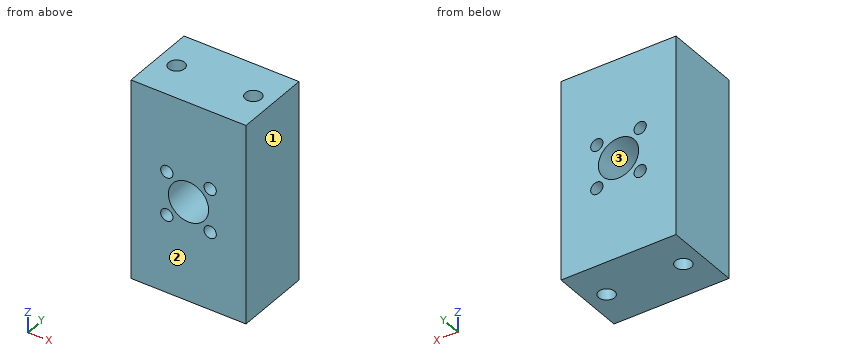
```python
from build123d import *

# Parameters (mm, degrees)
SKETCH_1_W          = 30
SKETCH_1_H          = 20
SKETCH_1_R          = 2.1
EXTRUDE_1_DEPTH     = 52
SKETCH_2_R          = 5.25
SKETCH_2_R_2        = 1.6
CUT_EXTRUDE_1_DEPTH = 64.277168078


with BuildPart() as part:
    # 草图1 → 凸台-拉伸1 (new body)
    with BuildSketch(Plane.XY):
        with Locations((15, 10)):
            Rectangle(SKETCH_1_W, SKETCH_1_H)
        with Locations(Location((5, 10, 0), (0, 0, 180))):
            Circle(SKETCH_1_R, mode=Mode.SUBTRACT)
        with Locations(Location((25, 10, 0), (0, 0, 180))):
            Circle(SKETCH_1_R, mode=Mode.SUBTRACT)
    extrude(amount=EXTRUDE_1_DEPTH)

    # 草图2 → 切除-拉伸1 (cut, through all)
    with BuildSketch(Plane(origin=(0, 20, 0), x_dir=(1, 0, 0), z_dir=(0, 1, 0))):
        with Locations(Location((15, -26, 0), (0, 0, 270))):
            Circle(SKETCH_2_R)
        with Locations(Location((9.343145751, -31.656854249, 0), (0, 0, 270))):
            Circle(SKETCH_2_R_2)
        with Locations(Location((9.343145751, -20.343145751, 0), (0, 0, 270))):
            Circle(SKETCH_2_R_2)
        with Locations(Location((20.656854249, -20.343145751, 0), (0, 0, 270))):
            Circle(SKETCH_2_R_2)
        with Locations(Location((20.656854249, -31.656854249, 0), (0, 0, 270))):
            Circle(SKETCH_2_R_2)
    extrude(amount=-CUT_EXTRUDE_1_DEPTH, mode=Mode.SUBTRACT)


solid = part.part
```
Input: part model. Units: mm. Frame: model coordinates. Face numbers are marked on the shaded views. Round coordinates to 2 decimals unless told otherwise and drop trailing zeros. Loops run counter-clockwise (first coordinate to the right, second up) from the corner with the lowest first, then second, coordinate; pieces in that order, holes last. Notation, with made-up numbers: (23, 2) -> (44, 2) arc R21 ccw to (44, 20) -> close; hole circle Ø11 at (-4, 6.5). An arc over 180 degrees is marked (long way). Use one line per item in the form item = value. Start each with the question number.
Item 1: Material intervals for L1, parallel to X at y = 10, z = 14; L2, parallel to X at y = 18.25, z = 31.5; L3, parallel to X at y = 14.25, z = 26, sorted ascending. Write a range as from..to.
Item 2: Contact query for a flat-ended pin moving along its axis: pin 1 Ø12 at (x, y) = (17.5, 6) entering from -Z. Output: stop coordinate, or through.
Item 3: Mould query, pull axis X, two halves, no side actions, for the marked faces 1, 2 and 3. Classes: pulls with the +X half, pulls with the -X half, needs draft (parallel to the pull), parting line crosses it, or undercut.
Item 4: Section query D-D on x = 15. Return the cut outline in (y, z).
Item 5: Section query A-A on x = 25. Return the cut outline in (y, z), then the cut area to 3 significant figures.
Item 6: Section query C-C on z = 17.5. Return the cut outline in (x, y), then the cut area to 3 significant figures.
Item 7: Section query B-B on z = 25. Return the cut outline in (x, y), then the cut area to 3 significant figures.
Ans:
q1.L1 = 0..2.9, 7.1..22.9, 27.1..30
q1.L2 = 0..7.75, 10.94..19.06, 22.25..30
q1.L3 = 0..9.75, 20.25..30
q2.pin_1 = 0
q3.face_1 = pulls with the +X half
q3.face_2 = needs draft
q3.face_3 = undercut
q4.outline = (0, 0) -> (20, 0) -> (20, 20.75) -> (0, 20.75) -> close; (0, 31.25) -> (20, 31.25) -> (20, 52) -> (0, 52) -> close
q5.outline = (0, 0) -> (7.9, 0) -> (7.9, 52) -> (0, 52) -> close; (12.1, 0) -> (20, 0) -> (20, 52) -> (12.1, 52) -> close
q5.area = 822 mm^2
q6.outline = (0, 0) -> (30, 0) -> (30, 20) -> (0, 20) -> close; hole circle Ø4.2 at (5, 10); hole circle Ø4.2 at (25, 10)
q6.area = 572 mm^2
q7.outline = (0, 0) -> (9.85, 0) -> (9.85, 20) -> (0, 20) -> close; (20.15, 0) -> (30, 0) -> (30, 20) -> (20.15, 20) -> close; hole circle Ø4.2 at (5, 10); hole circle Ø4.2 at (25, 10)
q7.area = 366 mm^2
